from build123d import *

# Parameters (mm, degrees)
SKETCH1_R           = 5
BOSS_EXTRUDE1_DEPTH = 3


with BuildPart() as part:
    # Sketch1 → Boss-Extrude1 (new body)
    with BuildSketch(Plane.XY):
        with BuildLine():
            ThreePointArc((0, 7.5), (-7.5, 0), (0, -7.5))
            ThreePointArc((0, -7.5), (60, -3.88694584), (120, -7.5))
            ThreePointArc((120, -7.5), (127.5, 0), (120, 7.5))
            ThreePointArc((120, 7.5), (60, 3.88694584), (0, 7.5))
        make_face()
        Circle(SKETCH1_R, mode=Mode.SUBTRACT)
        with Locations((120, 0)):
            Circle(SKETCH1_R, mode=Mode.SUBTRACT)
    extrude(amount=BOSS_EXTRUDE1_DEPTH)


solid = part.part
Geometry check sheet. Reference: the model listing, model coordinates, mm. Round coordinates to 2 decimals unless told otherwise and drop trailing zeros. Loops run counter-clockwise (first coordinate to the right, second up) from the corner with the lowest first, then second, coordinate; pieces in that order, holes last. Notation, with made-up numbers: (-19.5, 18.5) - (-1.5, 18.5) arc R21 cw to (-1.5, 24.5) - close; hole circle Ø7 at (9, 59.5). An arc over 180 degrees is marked (long way). One line per question, with ' | ' between items. Start each with the question number.
1. Depth check by flat-ended pin: pin 1 (1.5 mm diameter, centred on y = -4, z = 2, fed in from +X); pin 2 (1 mm diameter, centred on y = -4, z = 2, fed in from -X). Enter the tip coordinate at first touch or a pass-through.
2. Cross-section at D-D on x = 98. Record the cut outline in (y, z), then the cut area to 3 significant figures.
3. Scan lines: line 1 (X direction, y = -0.5, z = 2.2); line 2 (Y direction, x = 120, z = 1.8); line 3 (X direction, y = -1.5, z = 0.3). Record each from-to range of solid material in increasing order. Write a range as [from, to].
4. Draft check along Y on faces 1 (the face through (59.158, -3.888, 1.479)), 2 (the face through (127.5, -0.16, 1.48)), 3 (the face through (124.619, -1.915, 1.479)), 4 (the face through (59, 0, 3)). Enter one of: released by +Y, released by -Y, zero draft, split by the parting line, or undercut.
5. Cross-section at C-C on x = 31. Record the cut outline in (y, z).
6. Cross-section at B-B on z = 2.1. Record the cut outline in (x, y), then the cut area to 3 significant figures.
7. Cross-section at A-A on y = 0. Record the cut outline in (x, z), then the cut area to 3 significant figures.
Taken from the geometry:
1) pin 1: x = 126.76 | pin 2: x = -6.63
2) outline: (-5.33, 0) - (5.33, 0) - (5.33, 3) - (-5.33, 3) - close | area: 32.0 mm²
3) line 1: [-7.48, -4.97], [4.97, 115.03], [124.97, 127.48] | line 2: [-7.5, -5], [5, 7.5] | line 3: [-7.35, -4.77], [4.77, 115.23], [124.77, 127.35]
4) face 1: released by -Y | face 2: split by the parting line | face 3: undercut | face 4: zero draft
5) outline: (-4.73, 0) - (4.73, 0) - (4.73, 3) - (-4.73, 3) - close
6) outline: (0, -7.5) arc R500 cw to (120, -7.5) arc R7.5 ccw to (120, 7.5) arc R500 cw to (0, 7.5) arc R7.5 ccw to start; hole circle Ø10 at (0, 0); hole circle Ø10 at (120, 0) | area: 1,240 mm²
7) outline: (-7.5, 0) - (-5, 0) - (-5, 3) - (-7.5, 3) - close; (5, 0) - (115, 0) - (115, 3) - (5, 3) - close; (125, 0) - (127.5, 0) - (127.5, 3) - (125, 3) - close | area: 345 mm²
